```python
from build123d import *

# Parameters (mm, degrees)
SKETCH1_R               = 22.25
SKETCH1_R_2             = 8.5
SKETCH1_R_3             = 2.5
BOSS_EXTRUDE1_DEPTH     = 2.1
CUT_EXTRUDE2_DEPTH      = 32.536248984
CUT_EXTRUDE2_DEPTH_BACK = 32.536248984
SKETCH3_R               = 1.5


with BuildPart() as part:
    # Sketch1 → Boss-Extrude1 (new body)
    with BuildSketch(Plane.XY):
        Circle(SKETCH1_R)
        Circle(SKETCH1_R_2, mode=Mode.SUBTRACT)
        with Locations((17.75, 0)):
            Circle(SKETCH1_R_3, mode=Mode.SUBTRACT)
        with Locations((-17.75, 0)):
            Circle(SKETCH1_R_3, mode=Mode.SUBTRACT)
    extrude(amount=BOSS_EXTRUDE1_DEPTH)

    # Sketch3 → Cut-Extrude2 (cut, two sides: drawn at the far end of the back side and taken through both)
    with BuildSketch(Plane.XY.offset(-CUT_EXTRUDE2_DEPTH_BACK)):
        with Locations((4.508802817, -12.193059385)):
            Circle(SKETCH3_R)
        with Locations((4.508802817, 12.193059385)):
            Circle(SKETCH3_R)
        with Locations((-4.508802817, -12.193059385)):
            Circle(SKETCH3_R)
        with Locations((-4.508802817, 12.193059385)):
            Circle(SKETCH3_R)
    extrude(amount=CUT_EXTRUDE2_DEPTH + CUT_EXTRUDE2_DEPTH_BACK, mode=Mode.SUBTRACT)


solid = part.part
```
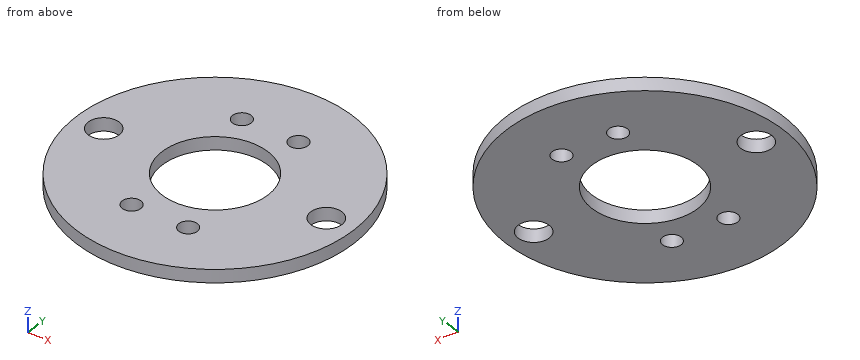
CAD build for the part. Positions are in the model's coordinates, mm. Coordinates: 2 decimals unless noted, no trailing zeros. Loops run counter-clockwise (first coordinate to the right, second up) from the corner with the lowest first, then second, coordinate; pieces in that order, holes last. Notation, with made-up numbers: (-31.75, 21) - (-11.75, 21) arc R21 cw to (-11.75, 57) - close; hole circle Ø11 at (11, 21). An arc over 180 degrees is marked (long way). Return JSON: item names as keys, results as strings.
1. Probe L1, parallel to X at y = -13, z = 0.75; L2, parallel to Y at x = 0, z = 1.35; L3, parallel to X at y = 3.5, z = 1.6. List the from-to ranges inside material, lowest first. Write a range as from..to.
Result:
{"L1": "x = -18.06..-5.77, -3.24..3.24, 5.77..18.06", "L2": "y = -22.25..-8.5, 8.5..22.25", "L3": "x = -21.97..-7.75, 7.75..21.97"}
2. Band-saw the part on A-A (x = 0). Give the cut face in (y, z), and give its area (4 significant figures).
Result:
{"outline": "(-22.25, 0) - (-8.5, 0) - (-8.5, 2.1) - (-22.25, 2.1) - close; (8.5, 0) - (22.25, 0) - (22.25, 2.1) - (8.5, 2.1) - close", "area": "57.75 mm2"}
3. Band-saw the part on D-D (x = 5.5). Give the cut face in (y, z), and give its area (3 significant figures).
Result:
{"outline": "(-21.56, 0) - (-13.32, 0) - (-13.32, 2.1) - (-21.56, 2.1) - close; (-11.07, 0) - (-6.48, 0) - (-6.48, 2.1) - (-11.07, 2.1) - close; (6.48, 0) - (11.07, 0) - (11.07, 2.1) - (6.48, 2.1) - close; (13.32, 0) - (21.56, 0) - (21.56, 2.1) - (13.32, 2.1) - close", "area": "53.9 mm2"}
4. Band-saw the part on B-B (y = -3.5). Give the cut face in (x, z), and give its area (3 significant figures).
Result:
{"outline": "(-21.97, 0) - (-7.75, 0) - (-7.75, 2.1) - (-21.97, 2.1) - close; (7.75, 0) - (21.97, 0) - (21.97, 2.1) - (7.75, 2.1) - close", "area": "59.8 mm2"}
5. Band-saw the part on C-C (y = -11.5). Give the cut face in (x, z).
Result:
{"outline": "(-19.05, 0) - (-5.84, 0) - (-5.84, 2.1) - (-19.05, 2.1) - close; (-3.18, 0) - (3.18, 0) - (3.18, 2.1) - (-3.18, 2.1) - close; (5.84, 0) - (19.05, 0) - (19.05, 2.1) - (5.84, 2.1) - close"}
